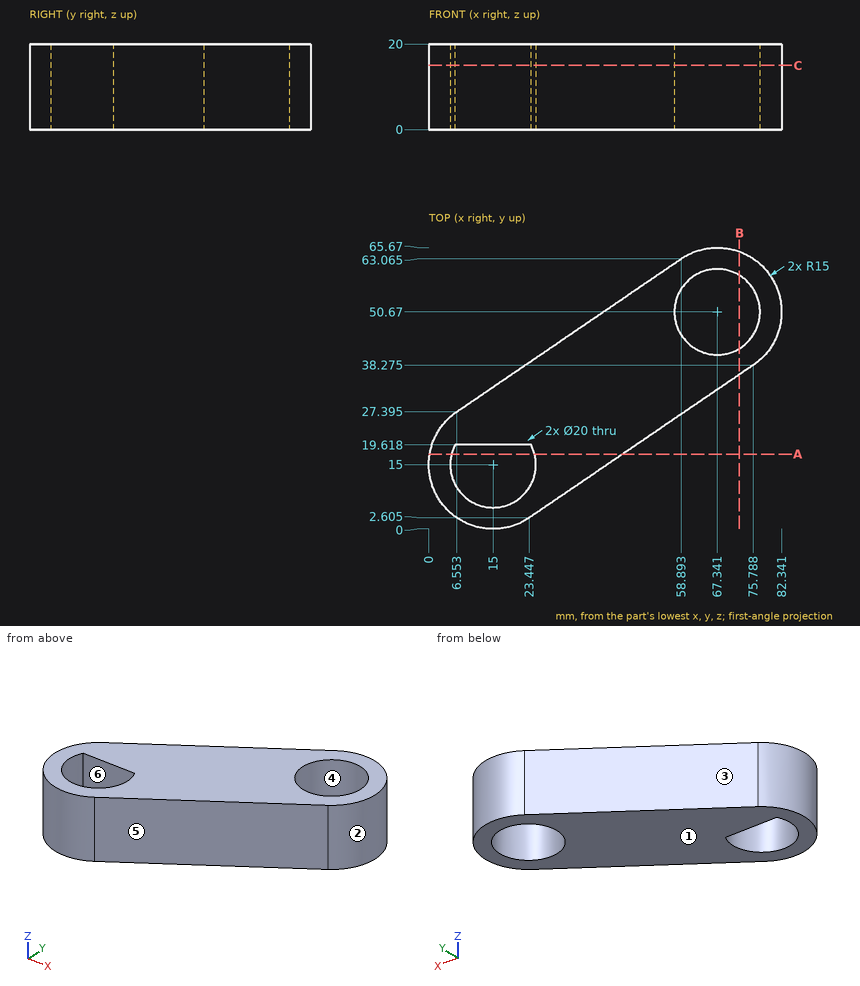
Geometry: see drawing. Coordinates: mm, zero at the bounding-box minimum. A direction names the side the tool comes from. Coordinates: 2 decimals unless noted, no trailing zeros. Order: outer loops, then holes, each group sorted by start corner. A loop starts at its lowest first (then second) coordinate and runs counter-clockwise, first axis right, second up. Notation, with made-up numbers: (83, 23.5) -> (131, 23.5) arc R16 cw to (131, 53.5) -> close; hole circle Ø8 at (61.5, -10.75). An arc over 180 degrees is marked (long way). Write each question's results on one line, items separated by ' | '. Start each with the question number.
1) Cut plane B-B, the plane x = 72.5. Output: boundary loops of the cut face in (y, z) (1 decimal), and give its area (3 significant figures).
2) Cut plane A-A, the plane y = 17.5. Output: boundary loops of the cut face in (x, z).
3) Mould query, pull axis Y, two halves, no side actions, for the marked faces 1, 2, 3 and 4. Classes: released by +Y, released by -Y, zero draft, split by the parting line, or undercut.
4) First-contact query: pin 1 (5 mm diameter, centred on x = 25.5, z = 7, fed in from -Y); pin 2 (1 mm diameter, centred on x = 12, z = 18, fed in from +Y); pin 3 (2 mm diameter, centred on y = 58, z = 9, fed in from +X); pin 4 (16 mm diameter, centred on x = 67.34, y = 50.67, fed in from -Z). Flat tips, straight axial feed; report the tip coordinate or a pass-through.
5) Cut plane C-C, the plane z = 15. Output: boundary loops of the cut face in (x, y) (1 decimal), and give its area (3 significant figures).
6) Set-up query: the marked faces 5 and 6. Return all of +Z, -Z, +X, -X, +Y, -Y with unobstructed straight access to the full face (end or side cutting, diameter ignored); none if empty.
7) Material intervals for line 1 along X through (y, z) = (8.5, 5.5) (1 decimal); line 2 along Y through (x, z) = (15, 12.25); line 3 along Y through (x, z) = (72, 12.25) (1 decimal), sorted ascending.
Checks:
1) outline: (36, 0) -> (42.1, 0) -> (42.1, 20) -> (36, 20) -> close; (59.2, 0) -> (64.8, 0) -> (64.8, 20) -> (59.2, 20) -> close | area: 232 mm^2
2) outline: (0.21, 0) -> (5.32, 0) -> (5.32, 20) -> (0.21, 20) -> close; (24.68, 0) -> (45.3, 0) -> (45.3, 20) -> (24.68, 20) -> close
3) face 1: zero draft | face 2: split by the parting line | face 3: released by +Y | face 4: undercut
4) pin 1: y = 2.31 | pin 2: y = 31.45 | pin 3: x = 80.94 | pin 4: through
5) outline: (6.6, 27.4) arc R15 ccw to (23.4, 2.6) -> (75.8, 38.3) arc R15 ccw to (58.9, 63.1) -> close; hole (6.1, 19.6) arc R10 ccw (long way) to (23.9, 19.6) -> close; hole circle Ø20 at (67.3, 50.7) | area: 2,050 mm^2
6) face 5: +Z, -Z, +X, -Y | face 6: +Z, -Z
7) line 1: 1.5 to 7.4, 22.6 to 32.1 | line 2: 0 to 5, 19.62 to 33.15 | line 3: 35.7 to 41.8, 59.5 to 64.9
